from build123d import *

# Parameters (mm, degrees)
BOSS_EXTRUDE1_DEPTH = 3
SKETCH2_W           = 480
SKETCH2_H           = 3
BOSS_EXTRUDE2_DEPTH = 20
SKETCH3_R           = 15.5
CUT_EXTRUDE1_DEPTH  = 0.2
SKETCH4_W           = 10
SKETCH4_H           = 3


with BuildPart() as part:
    # Sketch1 → Boss-Extrude1 (new body)
    with BuildSketch(Plane.XY):
        with BuildLine():
            Line((-240, -28.085620227), (-230, -28.085620227))
            ThreePointArc((-230, -28.085620227), (-201.715728753, -39.80134898), (-190, -68.085620227))
            Line((-190, -68.085620227), (-190, -135))
            ThreePointArc((-190, -135), (-160.710678119, -205.710678119), (-90, -235))
            Line((-90, -235), (90, -235))
            ThreePointArc((90, -235), (160.710678119, -205.710678119), (190, -135))
            Line((190, -135), (190, -68.085620227))
            ThreePointArc((190, -68.085620227), (201.715728753, -39.80134898), (230, -28.085620227))
            Line((230, -28.085620227), (240, -28.085620227))
            ThreePointArc((240, -28.085620227), (260, -8.085620227), (240, 11.914379773))
            Line((240, 11.914379773), (-240, 11.914379773))
            ThreePointArc((-240, 11.914379773), (-260, -8.085620227), (-240, -28.085620227))
        make_face()
    extrude(amount=BOSS_EXTRUDE1_DEPTH)

    # Sketch2 → Boss-Extrude2 (add)
    with BuildSketch(Plane.XY.offset(3)):
        with Locations((0, 10.414379773)):
            Rectangle(SKETCH2_W, SKETCH2_H)
    extrude(amount=BOSS_EXTRUDE2_DEPTH)

    # Sketch3 → Cut-Extrude1 (cut)
    with BuildSketch(Plane.XY.offset(3)):
        with Locations((-240, -8.085620227)):
            Circle(SKETCH3_R)
        with Locations(Location((240, -8.085620227, 0), (0, 0, 180))):
            Circle(SKETCH3_R)
    extrude(amount=-CUT_EXTRUDE1_DEPTH, mode=Mode.SUBTRACT)

    # Sweep1: sweep along a path in Sketch5
    with BuildLine(Plane.XY.offset(3)) as sweep1_path:
        ThreePointArc((-240, 11.914379773), (-260, -8.085620227), (-240, -28.085620227))
        Line((-240, -28.085620227), (-230, -28.085620227))
        ThreePointArc((-230, -28.085620227), (-201.715728753, -39.80134898), (-190, -68.085620227))
        Line((-190, -68.085620227), (-190, -135))
        ThreePointArc((-190, -135), (-160.710678119, -205.710678119), (-90, -235))
        Line((-90, -235), (90, -235))
        ThreePointArc((90, -235), (160.710678119, -205.710678119), (190, -135))
        Line((190, -135), (190, -68.085620227))
        ThreePointArc((190, -68.085620227), (201.715728753, -39.80134898), (230, -28.085620227))
        Line((230, -28.085620227), (240, -28.085620227))
        ThreePointArc((240, -28.085620227), (260, -8.085620227), (240, 11.914379773))
    # Sketch4 → Sweep1 (sweep)
    with BuildSketch(Plane.ZY.offset(240)):
        with Locations((8, 10.414379773)):
            Rectangle(SKETCH4_W, SKETCH4_H)
    sweep(path=sweep1_path.line)


solid = part.part
Here's how the part is built. I have some questions about the finished solid (model axes, mm). A direction names the side the tool comes from. Give positions to 0.01 mm unless a question says otherwise; leave off trailing zeros. Loops run counter-clockwise (first coordinate to the right, second up) from the corner with the lowest first, then second, coordinate; pieces in that order, holes last. Notation, with made-up numbers: (77, -4) -> (136, -4) arc R24 ccw to (136, 24) -> close; hole circle Ø2 at (63, 55). An arc over 180 degrees is marked (long way). Answer as a JSON object with one key per item and string values. Group by question number.
Item 1: Imagine slicing it at B-B on y = -87.5. Write out the boundary of the cut face in (x, z), then the cut area to 3 significant figures.
Item 2: I need wall thicknesses on L1, parallel to Y at x = 85.5, z = 11.25; L2, parallel to Y at x = 240, z = 2.95; L3, parallel to X at y = -79, z = 10.5. Which ranges of each line are inside material? Lowest first, please.
Item 3: Will these pins go through, and if not, where does the flat tip stop? pin 1 (1.5 mm diameter, centred on x = 99, z = 8, fed in from -Y); pin 2 (8 mm diameter, centred on x = -176.5, z = 13.5, fed in from -Y); pin 3 (10.5 mm diameter, centred on y = -89, z = 9.5, fed in from +X); pin 4 (10 mm diameter, centred on x = -185.5, y = -51, fed in from -Z).
Item 4: Thinking about a two-plate mould opening in X: for faces 5 (the flat face through (-4, -110, 0)), 6 (the flat face through (1, -232, 8)), 7 (the cylindrical face through (201.41, -40.11, 6.41)), which applies, pulls with the +X half, pulls with the -X half, needs draft (parallel to the pull), parting line crosses it, or undercut?
Item 5: Imagine slicing it at A-A on z = 8.5. Write out the boundary of the cut face in (x, y), then the cut area to 3 significant figures.
Item 6: Imagine slicing it at C-C on y = -43. Write out the boundary of the cut face in (x, z).
Item 7: On a 3-axis mill with a long thin cutter (end or side, diameter ignored), from which of +Z, -Z, +X, -X, +Y, -Y can I reach the whole of each face in a straight line? I mean faces 1 (the flat face through (-3, 11.914, 11)), 2 (the flat face through (235, -28.086, 7)), 3 (the flat face through (-190, -102, 7)), 4 (the cylindrical face through (-199.93, -37.35, 8.07)). Say none if no direction works.
Answer list:
{
 "1": {"outline": "(-190, 0) -> (190, 0) -> (190, 13) -> (187, 13) -> (187, 3) -> (-187, 3) -> (-187, 13) -> (-190, 13) -> close", "area": "1,200 mm2"},
 "2": {"L1": "y = -235 to -232, 8.91 to 11.91", "L2": "y = -28.09 to -23.59, 7.41 to 11.91", "L3": "x = -190 to -187, 187 to 190"},
 "3": {"pin 1": "stops at y = -234.66", "pin 2": "stops at y = -191.47", "pin 3": "stops at x = 190", "pin 4": "stops at z = 0"},
 "4": {"face 5": "needs draft", "face 6": "undercut", "face 7": "pulls with the +X half"},
 "5": {"outline": "(-240, -28.09) -> (-230, -28.09) arc R40 cw to (-190, -68.09) -> (-190, -135) arc R100 ccw to (-90, -235) -> (90, -235) arc R100 ccw to (190, -135) -> (190, -68.09) arc R40 cw to (230, -28.09) -> (240, -28.09) arc R20 ccw to (240, 11.91) -> (-240, 11.91) arc R20 ccw to start; hole (-240, -25.09) -> (-230, -25.09) arc R43 cw to (-187, -68.09) -> (-187, -135) arc R97 ccw to (-90, -232) -> (90, -232) arc R97 ccw to (187, -135) -> (187, -68.09) arc R43 cw to (230, -25.09) -> (240, -25.09) arc R17 ccw to (240, 8.91) -> (-240, 8.91) arc R17 ccw to start", "area": "4,110 mm2"},
 "6": {"outline": "(-198.84, 0) -> (198.84, 0) -> (198.84, 13) -> (195.08, 13) -> (195.08, 3) -> (-195.08, 3) -> (-195.08, 13) -> (-198.84, 13) -> close"},
 "7": {"face 1": "+Z, -Z, +X, -X, +Y", "face 2": "+Z, -Z, +X, -Y", "face 3": "+Z, -Z, -X, -Y", "face 4": "+Z"}
}
